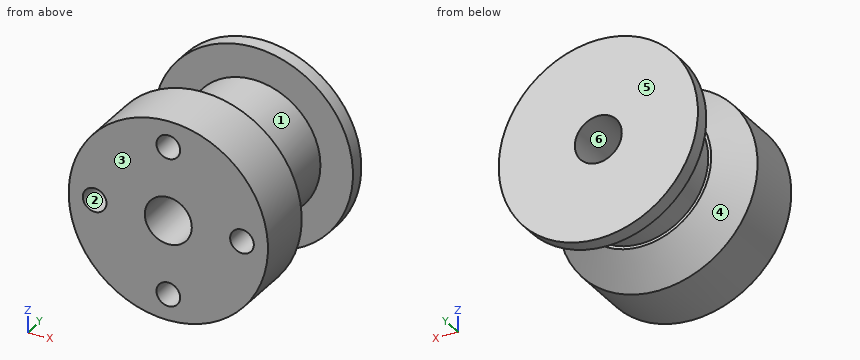
from build123d import *

# Parameters (mm, degrees)
CHAMFER1_SIZE             = 2
M2X0_4_TAPPED_HOLE1_D     = 1.6
M2X0_4_TAPPED_HOLE1_DEPTH = 3
M2X0_4_TAPPED_HOLE1_TIP   = 0.480688495


with BuildPart() as part:
    # Sketch1 → Revolve1 (revolve)
    with BuildSketch(Plane.XY, mode=Mode.PRIVATE) as revolve1_sk:
        Polygon((1.5875, 0), (1.5875, 11.1252), (6.73, 11.1252), (6.73, 10.1252), (4.5339, 10.1252), (4.5339, 6.019800098), (6.731, 6.019800098), (6.731, 0), align=None)
    revolve(revolve1_sk.sketch.rotate(Axis((0, 0, 0), (0, 1, 0)), 90), axis=Axis((0, 0, 0), (0, 1, 0)))

    # Chamfer1
    chamfer1_edges = [part.edges().sort_by_distance(p)[0] for p in [
        (0, 6.019800098, 6.731),
    ]]
    chamfer(chamfer1_edges, length=CHAMFER1_SIZE)

    # M2x0.4 Tapped Hole1
    with Locations(Plane(origin=(0, 0, 0), x_dir=(-1, 0, 0), z_dir=(0, -1, 0))):
        with Locations((0, -4.977300526), (-4.977300526, 0), (0, 4.977300526), (4.977300526, 0), (0, 0)):
            Hole(M2X0_4_TAPPED_HOLE1_D / 2, depth=M2X0_4_TAPPED_HOLE1_DEPTH)
            with Locations((0, 0, -(M2X0_4_TAPPED_HOLE1_DEPTH + M2X0_4_TAPPED_HOLE1_TIP / 2))):  # 118° drill point
                Cone(0, M2X0_4_TAPPED_HOLE1_D / 2, M2X0_4_TAPPED_HOLE1_TIP, mode=Mode.SUBTRACT)


solid = part.part
Here's how the part is built. I have some questions about the finished solid (model axes, mm). Face numbers are marked on the shaded views. A direction names the side the tool comes from. Give positions to 0.01 mm unless a question says otherwise; leave off trailing zeros. Loops run counter-clockwise (first coordinate to the right, second up) from the corner with the lowest first, then second, coordinate; pieces in that order, holes last. Notation, with made-up numbers: (-13.75, 79.5) -> (0.25, 79.5) arc R30 ccw to (0.25, 112.5) -> close; hole circle Ø1 at (16, 85). An arc over 180 degrees is marked (long way). Answer as a JSON object with one key per item and string values. Group by question number.
Item 1: Imagine slicing it at A-A on y = 9.25. Write out the boundary of the cut face in (x, z) (1 decimal).
Item 2: Will these pins go through, and if not, where does the flat tip stop? pin 1 (3 mm diameter, centred on x = -1.5, y = 7, fed in from -Z); pin 2 (6 mm diameter, centred on y = 1.5, z = -4, fed in from +X); pin 3 (3 mm diameter, centred on x = 0, z = 0, fed in from -Y); pin 4 (1.5 mm diameter, centred on x = 1, y = 3.5, fed in from +Z).
Item 3: I need wall thicknesses on L1, parallel to X at y = 7, z = 0; L2, parallel to Z at x = 0.5, y = 0.75; L3, parallel to Y at x = 6, z = 2.25. Which ranges of each line are inside material? Lowest first, please.
Item 4: On a 3-axis mill with a long thin cutter (end or side, diameter ignored), from which of +Z, -Z, +X, -X, +Y, -Y can I reach the whole of each face in a straight line? I mean the marked faces 1, 2 and 3. Say none if no direction works.
Item 5: Imagine slicing it at B-B on y = 4.75. Write out the boundary of the cut face in (x, z) (1 decimal), then the cut area to 3 significant figures.
Item 6: Thinking about a two-plate mould opening in Y: for the marked faces 4, 5 and 6, which applies, pulls with the +Y half, pulls with the -Y half, needs draft (parallel to the pull), parting line crosses it, or undercut?
Answer list:
{
 "1": {"outline": "circle Ø9.1 at (0, 0); hole circle Ø3.2 at (0, 0)"},
 "2": {"pin 1": "stops at z = -5.08", "pin 2": "stops at x = 6.66", "pin 3": "passes through", "pin 4": "stops at z = 6.73"},
 "3": {"L1": "x = -4.53 to -1.59, 1.59 to 4.53", "L2": "z = -6.71 to -5.6, -4.35 to -1.51, 1.51 to 4.35, 5.6 to 6.71", "L3": "y = 0 to 4.34, 10.13 to 11.13"},
 "4": {"face 1": "none", "face 2": "-Y", "face 3": "+Z, -Z, +X, -X, -Y"},
 "5": {"outline": "circle Ø12 at (0, 0); hole circle Ø3.2 at (0, 0)", "area": "105 mm2"},
 "6": {"face 4": "undercut", "face 5": "pulls with the +Y half", "face 6": "needs draft"}
}
